For this review, take the finished solid that the model builds, in its own axes (mm). A direction names the side the tool comes from. Give positions to 0.01 mm unless a question says otherwise; leave off trailing zeros. Write each loop counter-clockwise with the first axis right and the second up, starting at its lowest first coordinate (ties: lowest second). Pieces come first, ordered by that corner, then holes. Notation, with made-up numbers: (69.5, 37.25) -> (92.5, 37.25) arc R18 ccw to (92.5, 45.25) -> close; hole circle Ø10 at (6.25, -5.75). An arc over 180 degrees is marked (long way). Write item = value, one per line.
```python
from build123d import *

# Parameters (mm, degrees)
CROQUIS1_R              = 10.5
SALIENTE_EXTRUIR1_DEPTH = 2
CROQUIS2_R              = 4
CROQUIS2_R_2            = 2
SALIENTE_EXTRUIR2_DEPTH = 3
REDONDEO1_R             = 1
CROQUIS3_R              = 4
CROQUIS3_R_2            = 3
CORTAR_EXTRUIR1_DEPTH   = 1
CROQUIS4_R              = 2
CORTAR_EXTRUIR2_DEPTH   = 3
CROQUIS5_R              = 2.5
CORTAR_EXTRUIR3_DEPTH   = 1
CROQUIS6_R              = 0.6
CORTAR_EXTRUIR4_DEPTH   = 6
MATRIZC1_COUNT          = 4
REDONDEO2_R             = 0.2


with BuildPart() as part:
    # Croquis1 → Saliente-Extruir1 (new body)
    with BuildSketch(Plane(origin=(0, 0, 0), x_dir=(1, 0, 0), z_dir=(0, 1, 0))):
        Circle(CROQUIS1_R)
    extrude(amount=SALIENTE_EXTRUIR1_DEPTH)

    # Croquis2 → Saliente-Extruir2 (add)
    with BuildSketch(Plane.XZ):
        Circle(CROQUIS2_R)
        Circle(CROQUIS2_R_2, mode=Mode.SUBTRACT)
    extrude(amount=SALIENTE_EXTRUIR2_DEPTH)

    # Redondeo1
    redondeo1_edges = [part.edges().sort_by_distance(p)[0] for p in [
        (-4, -3, 0),
    ]]
    fillet(redondeo1_edges, radius=REDONDEO1_R)

    # Croquis3 → Cortar-Extruir1 (cut)
    with BuildSketch(Plane(origin=(0, 2, 0), x_dir=(1, 0, 0), z_dir=(0, 1, 0))):
        Circle(CROQUIS3_R)
        Circle(CROQUIS3_R_2, mode=Mode.SUBTRACT)
    extrude(amount=-CORTAR_EXTRUIR1_DEPTH, mode=Mode.SUBTRACT)

    # Croquis4 → Cortar-Extruir2 (cut)
    with BuildSketch(Plane(origin=(0, 2, 0), x_dir=(1, 0, 0), z_dir=(0, 1, 0))):
        Circle(CROQUIS4_R)
    extrude(amount=-CORTAR_EXTRUIR2_DEPTH, mode=Mode.SUBTRACT)

    # Croquis5 → Cortar-Extruir3 (cut)
    with BuildSketch(Plane(origin=(0, 2, 0), x_dir=(1, 0, 0), z_dir=(0, 1, 0))):
        Circle(CROQUIS5_R)
    extrude(amount=-CORTAR_EXTRUIR3_DEPTH, mode=Mode.SUBTRACT)

    # Croquis6 → Cortar-Extruir4 (cut, through all)
    with BuildSketch(Plane(origin=(0, 2, 0), x_dir=(1, 0, 0), z_dir=(0, 1, 0))):
        with Locations((0, 7.25)):
            Circle(CROQUIS6_R)
        with Locations((3.5, 7.25)):
            Circle(CROQUIS6_R)
        with Locations((-3.5, 7.25)):
            Circle(CROQUIS6_R)
    cortar_extruir4 = extrude(amount=-CORTAR_EXTRUIR4_DEPTH, mode=Mode.SUBTRACT)

    # MatrizC1: Cortar-Extruir4 ×4 about axis
    matrizc1_axis = Axis((0, 0, 0), (0, 1, 0))
    for i in range(1, MATRIZC1_COUNT):
        add(cortar_extruir4.rotate(matrizc1_axis, i * 360 / MATRIZC1_COUNT), mode=Mode.SUBTRACT)

    # Redondeo2
    redondeo2_edges = [part.edges().sort_by_distance(p)[0] for p in [
        (-4, 2, 0),
        (-3, 2, 0),
        (-2.5, 2, 0),
    ]]
    fillet(redondeo2_edges, radius=REDONDEO2_R)


solid = part.part
```
(1) Take a section at D-D (x = -7.25). Write out the cut boundary in (y, z).
Answers below:
outline = (0, -7.6) -> (2, -7.6) -> (2, -4.1) -> (0, -4.1) -> close; (0, -2.9) -> (2, -2.9) -> (2, -0.6) -> (0, -0.6) -> close; (0, 0.6) -> (2, 0.6) -> (2, 2.9) -> (0, 2.9) -> close; (0, 4.1) -> (2, 4.1) -> (2, 7.6) -> (0, 7.6) -> close
(2) Take a section at B-B (z = 7.25). Write out the cut boundary in (x, y).
Answers below:
outline = (-7.6, 0) -> (-4.1, 0) -> (-4.1, 2) -> (-7.6, 2) -> close; (-2.9, 0) -> (-0.6, 0) -> (-0.6, 2) -> (-2.9, 2) -> close; (0.6, 0) -> (2.9, 0) -> (2.9, 2) -> (0.6, 2) -> close; (4.1, 0) -> (7.6, 0) -> (7.6, 2) -> (4.1, 2) -> close
(3) Tool access review of faces 5 (the face through (-0.54, 1.41, 2.44)), 6 (the face through (10, 1, -3.2)): name each direction out of +Z, -Z, +X, -X, +Y, -Y from which nothing blocks a thin tool from reaching the whole face with its end or side.
Answers below:
face_5 = +Y
face_6 = +Y, -Y
(4) For pin 1 (3 mm diameter, centred on x = -1, z = -8.5, fed in from -Y); pin 2 (2 mm diameter, centred on y = 0, z = -7.5, fed in from +X); pin 3 (3 mm diameter, centred on y = 0, z = 6.5, fed in from +X), all flat-tipped, find the tip position at first contact; note any pin that passes through.
Answers below:
pin_1 = 0
pin_2 = 8.25
pin_3 = 9.23
(5) The part is to be moulded in two halves that separate along Z. For faces 1 (the face through (5, 0, 0)), 2 (the face through (-0.867, -0.986, -3.905)), 3 (the face through (0.13, 1.014, 6.664)), 4 (the face through (6.664, 1.014, 3.37)), say which applies: released by +Z, released by -Z, zero draft, split by the parting line, or undercut.
Answers below:
face_1 = zero draft
face_2 = split by the parting line
face_3 = undercut
face_4 = undercut
(6) To check wall thickness, follow probe 1 along Z at (x, y) = (0, 1.4); probe 2 along X at (y, z) = (0.75, 0); probe 3 along Z at (x, y) = (-7.25, 0.85). State the ranges of each line that lie inside material, in increasing order.
Answers below:
probe_1 = -10.5 to -7.85, -6.65 to -4, -3 to -2.5, 2.5 to 3, 4 to 6.65, 7.85 to 10.5
probe_2 = -10.5 to -7.85, -6.65 to -2, 2 to 6.65, 7.85 to 10.5
probe_3 = -7.6 to -4.1, -2.9 to -0.6, 0.6 to 2.9, 4.1 to 7.6
(7) Take a section at A-A (y = 1.55). Count the separate pieces of the cut face and the enclosed holes in it, plus the area to 3 significant figures.
Answers below:
separate_pieces = 2
enclosed_holes = 14
area = 291 mm^2
